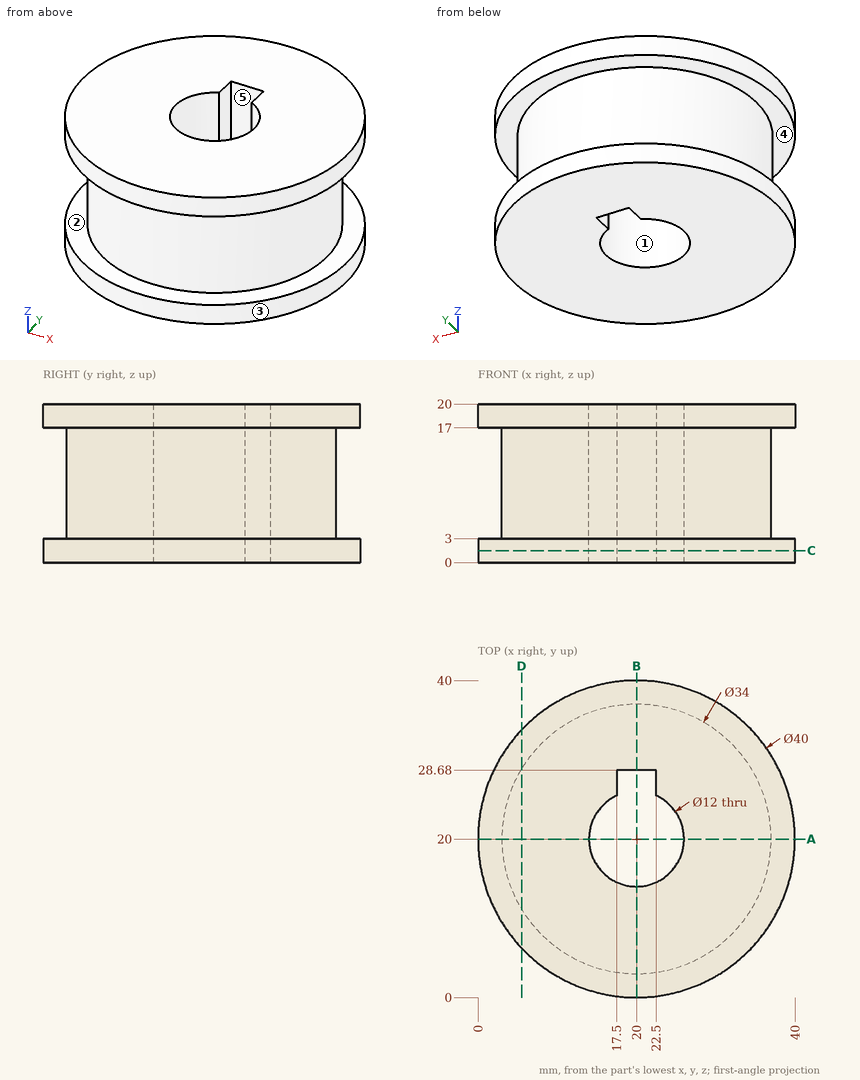
Geometry check sheet. Reference: drawing and pictorial views, mm from the part's lowest x, y, z. A direction names the side the tool comes from. Give positions to 0.01 mm unless a question says otherwise; leave off trailing zeros. Loops run counter-clockwise (first coordinate to the right, second up) from the corner with the lowest first, then second, coordinate; pieces in that order, holes last.
1. Thickness scan on line 1 (Y direction, x = 20, z = 12); line 2 (Z direction, x = 35, y = 33); line 3 (Y direction, x = 21, z = 11.75). Record the ranges inside material, lowest first.
2. Go/stop test with flat-tipped pins: pin 1 Ø3 at (x, z) = (34.5, 9.5) entering from -Y; pin 2 Ø8 at (x, z) = (34, 13.5) entering from -Y; pin 3 Ø1.5 at (x, z) = (34.5, 4) entering from +Y. Record where each tip stops, or that it passes through.
3. Set-up check for the marked faces 1 and 2: record each of +Z, -Z, +X, -X, +Y, -Y from which the full face is reachable in a straight line by a thin tool's end or side.
4. Section check D-D, the plane x = 5.5. Enter the section's corners in (y, z), then the cut area to 3 significant figures.
5. Mould release check, pull along Y, two halves, no side actions. Record for the marked faces 3, 4 and 5: released by +Y, released by -Y, zero draft, split by the parting line, or undercut.
6. Section check C-C, the plane z = 1.5. Enter the section's corners in (x, y), then the cut area to 3 significant figures.
7. Section check A-A, the plane y = 20. Enter the section's corners in (x, z), then the cut area to 3 significant figures.
8. Section check B-B, the plane x = 20. Enter the section's corners in (y, z), then the cut area to 3 significant figures.
Geometry says:
1. line 1: y = 3 to 14, 28.68 to 37
1. line 2: z = 0 to 3, 17 to 20
1. line 3: y = 3.03 to 14.08, 28.68 to 36.97
2. pin 1: stops at y = 9.05
2. pin 2: stops at y = 4.05
2. pin 3: stops at y = 30
3. face 1: +Z, -Z
3. face 2: none
4. outline: (6.23, 0) - (33.77, 0) - (33.77, 3) - (28.87, 3) - (28.87, 17) - (33.77, 17) - (33.77, 20) - (6.23, 20) - (6.23, 17) - (11.13, 17) - (11.13, 3) - (6.23, 3) - close
4. area: 414 mm2
5. face 3: split by the parting line
5. face 4: zero draft
5. face 5: undercut
6. outline: circle Ø40 at (20, 20); hole (17.5, 25.45) arc R6 ccw (long way) to (22.5, 25.45) - (22.5, 28.68) - (17.5, 28.68) - close
6. area: 1,130 mm2
7. outline: (0, 0) - (14, 0) - (14, 20) - (0, 20) - (0, 17) - (3, 17) - (3, 3) - (0, 3) - close; (26, 0) - (40, 0) - (40, 3) - (37, 3) - (37, 17) - (40, 17) - (40, 20) - (26, 20) - close
7. area: 476 mm2
8. outline: (0, 0) - (14, 0) - (14, 20) - (0, 20) - (0, 17) - (3, 17) - (3, 3) - (0, 3) - close; (28.68, 0) - (40, 0) - (40, 3) - (37, 3) - (37, 17) - (40, 17) - (40, 20) - (28.68, 20) - close
8. area: 422 mm2
